Part print with two shaded views. Sizes in mm from the minimum x, y, z corner. Give positions to 0.01 mm unless a question says otherwise; leave off trailing zeros. Write each loop counter-clockwise with the first axis right and the second up, starting at its lowest first coordinate (ties: lowest second). Pieces come first, ordered by that corner, then holes. Notation, with made-up numbers: (-38.75, -33) -> (6.25, -33) arc R31 ccw to (6.25, -7) -> close; hole circle Ø9 at (-29, 78.5). An arc over 180 degrees is marked (long way). Write item = value, one per line. Start each with the question number.
Q1. Saw through at B-B, the plane y = 5.75. List the corners of the cut face in (x, z) (1 decimal).
Q2. Saw through at D-D, the plane y = 6.75. List the corners of the cut face in (x, z) (1 decimal).
Q3. Wall check: line 1 (Z direction, x = 0.55, y = 1.25); line 2 (Y direction, x = 0.25, z = 4.5); line 3 (Z direction, x = 0.2, y = 4). Give the ranges that are in metal, low to high.
Q4. Drop a flat-ended pin along its axis: P1, Ø1.5, axis at y = 3.5, z = 5, coming from the -X side. Give the stop position or say it passes through.
Q5. Saw through at C-C, the plane z = 1.75. List the corners of the cut face in (x, y) (1 decimal).
Q6. Mould opens along Y. For the marked faces 1, 2 and 3 say: pulls with the +Y half, pulls with the -Y half, needs draft (parallel to the pull), parting line crosses it, or undercut.
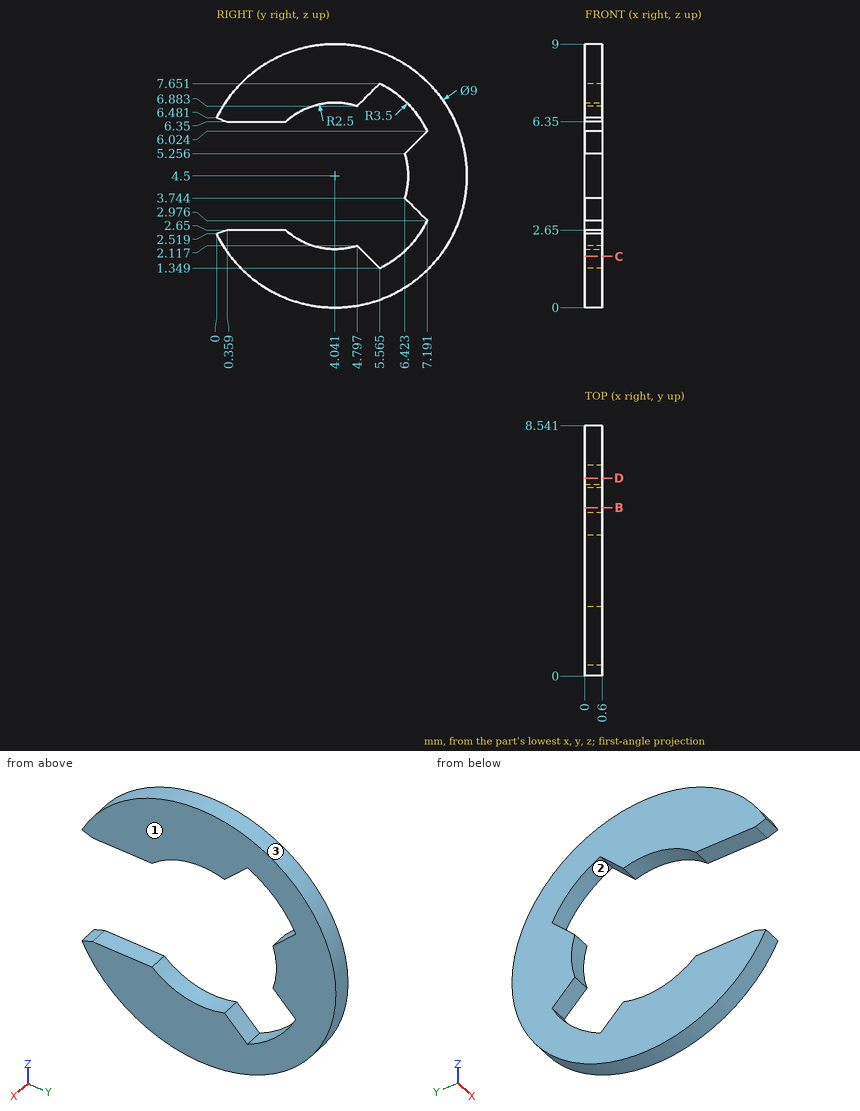
Report:
q1.outline = (0, 0.3) -> (0.6, 0.3) -> (0.6, 1.4) -> (0, 1.4) -> close; (0, 7.6) -> (0.6, 7.6) -> (0.6, 8.7) -> (0, 8.7) -> close
q2.outline = (0, 0.9) -> (0.6, 0.9) -> (0.6, 2.3) -> (0, 2.3) -> close; (0, 3.4) -> (0.6, 3.4) -> (0.6, 5.6) -> (0, 5.6) -> close; (0, 6.7) -> (0.6, 6.7) -> (0.6, 8.1) -> (0, 8.1) -> close
q3.line_1 = 0.97 to 2.65, 6.35 to 8.03
q3.line_2 = 6.54 to 8.54
q3.line_3 = 0 to 2, 7 to 9
q4.P1 = through
q5.outline = (0, 0.5) -> (0.6, 0.5) -> (0.6, 5.2) -> (0, 5.2) -> close; (0, 6.2) -> (0.6, 6.2) -> (0.6, 7.6) -> (0, 7.6) -> close
q6.face_1 = needs draft
q6.face_2 = undercut
q6.face_3 = parting line crosses it
